from build123d import *

# Parameters (mm, degrees)
SKETCH_1_R      = 3.8
SKETCH_1_R_2    = 2.525
EXTRUDE_1_DEPTH = 2.75
FILLET_1_R      = 0.1


with BuildPart() as part:
    # Эскиз1 → Бобышка-Вытянуть1 (new body)
    with BuildSketch(Plane(origin=(0, 0, 0), x_dir=(1, 0, 0), z_dir=(0, 1, 0))):
        Circle(SKETCH_1_R)
        Circle(SKETCH_1_R_2, mode=Mode.SUBTRACT)
    extrude(amount=EXTRUDE_1_DEPTH)

    # Скругление1
    fillet_1_edges = [part.edges().sort_by_distance(p)[0] for p in [
        (-3.8, 0, 0),
        (-3.8, 2.75, 0),
        (-2.525, 0, 0),
        (-2.525, 2.75, 0),
    ]]
    fillet(fillet_1_edges, radius=FILLET_1_R)


solid = part.part
Source: CAD feature listing. Evaluate the final solid. Frame: model axes, mm. Coordinates: 2 decimals unless noted, no trailing zeros. Order: outer loops, then holes, each group sorted by start corner. A loop starts at its lowest first (then second) coordinate and runs counter-clockwise, first axis right, second up.
Item 1: Cut plane A-A (z = 0). Return loops of the section in (x, y) (3 decimals).
Output values:
outline: (-3.8, 0.1) arc R0.1 ccw to (-3.7, 0) - (-2.625, 0) arc R0.1 ccw to (-2.525, 0.1) - (-2.525, 2.65) arc R0.1 ccw to (-2.625, 2.75) - (-3.7, 2.75) arc R0.1 ccw to (-3.8, 2.65) - close; (2.525, 0.1) arc R0.1 ccw to (2.625, 0) - (3.7, 0) arc R0.1 ccw to (3.8, 0.1) - (3.8, 2.65) arc R0.1 ccw to (3.7, 2.75) - (2.625, 2.75) arc R0.1 ccw to (2.525, 2.65) - close
Item 2: Cut plane C-C (y = 2.3). Return loops of the section in (x, z) (3 decimals), plus the area to 3 significant figures.
Output values:
outline: circle Ø7.6 at (0, 0); hole circle Ø5.05 at (0, 0)
area: 25.3 mm2
Item 3: First-contact query: P1, Ø1, axis at y = 2, z = -2.5, coming from the +X side. Flat tip, straight axial feed; report the tip coordinate or a pass-through.
Output values:
P1: stops at x = 3.23
Item 4: Pull-direction query (X, two-part tool) for faces 1 (the face through (1, 2.75, -3)), 2 (the face through (-3.796, 1.357, -0.167)), 3 (the face through (2.41, 1.36, -0.76)); classes: pulls with the +X half, pulls with the -X half, needs draft (parallel to the pull), parting line crosses it, or undercut.
Output values:
face 1: needs draft
face 2: parting line crosses it
face 3: undercut
Item 5: Material intervals for line 1 (X direction, y = 1.3, z = 0) (3 decimals); line 2 (X direction, y = 1.35, z = -2.25), sorted ascending.
Output values:
line 1: x = -3.8 to -2.525, 2.525 to 3.8
line 2: x = -3.06 to -1.15, 1.15 to 3.06
Item 6: Cut plane B-B (x = 0). Return loops of the section in (y, z) (3 decimals), plus the area to 3 significant figures.
Output values:
outline: (0, -3.7) arc R0.1 ccw to (0.1, -3.8) - (2.65, -3.8) arc R0.1 ccw to (2.75, -3.7) - (2.75, -2.625) arc R0.1 ccw to (2.65, -2.525) - (0.1, -2.525) arc R0.1 ccw to (0, -2.625) - close; (0, 2.625) arc R0.1 ccw to (0.1, 2.525) - (2.65, 2.525) arc R0.1 ccw to (2.75, 2.625) - (2.75, 3.7) arc R0.1 ccw to (2.65, 3.8) - (0.1, 3.8) arc R0.1 ccw to (0, 3.7) - close
area: 7.00 mm2
